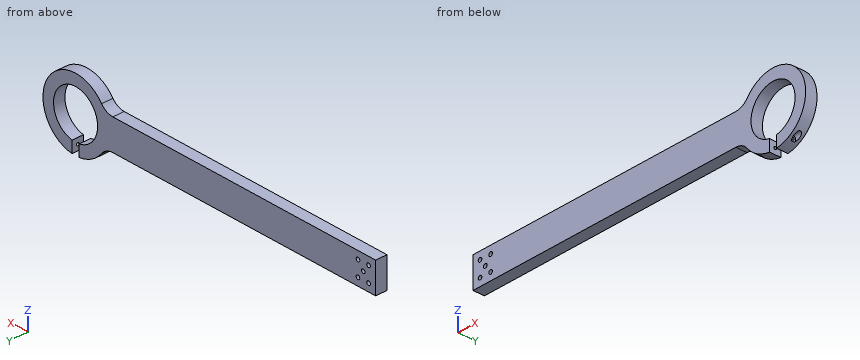
from build123d import *

# Parameters (mm, degrees)
BOSS_EXTRUDE1_DEPTH   = 4.7625
SKETCH8_W             = 1.1303
SKETCH8_H             = 266.825
F_4_40_TAPPED_HOLE2_D = 2.2606
FILLET2_R             = 12.7
CUT_EXTRUDE1_START    = -9.525
SKETCH11_R            = 2.413
CUT_EXTRUDE1_DEPTH    = 17.6497001
F_4_CLEARANCE_HOLE1_D = 3.2639


with BuildPart() as part:
    # Sketch2 → Boss-Extrude1 (new body, symmetric)
    with BuildSketch(Plane(origin=(0, 0, 0), x_dir=(1, 0, 0), z_dir=(0, 1, 0))):
        with BuildLine():
            Line((266.825, 19.568804386), (266.825, 29.177461594))
            ThreePointArc((266.825, 29.177461594), (253.046230135, 23.957766537), (243.54031576, 12.7))
            Line((243.54031576, 12.7), (0, 12.7))
            Line((0, 12.7), (0, -12.7))
            Line((0, -12.7), (243.54031576, -12.7))
            ThreePointArc((243.54031576, -12.7), (293.957766537, -16.953769865), (273.175, 29.177461594))
            Line((273.175, 29.177461594), (273.175, 19.568804386))
            ThreePointArc((273.175, 19.568804386), (270, -19.8247), (266.825, 19.568804386))
        make_face()
    extrude(amount=BOSS_EXTRUDE1_DEPTH, both=True)

    # Sketch8 → #4-40 Tapped Hole1 (revolve, cut)
    with BuildSketch(Plane(origin=(266.825, 0, -24.37313299), x_dir=(0, 0, -1), z_dir=(0, 1, 0))):
        with Locations((0.56515, 133.4125)):
            Rectangle(SKETCH8_W, SKETCH8_H)
    revolve(axis=Axis((273.175, 0, -24.37313299), (-1, 0, 0)), mode=Mode.SUBTRACT)

    # #4-40 Tapped Hole2 (through all)
    with Locations(Plane.ZY.offset(-273.175)):
        with Locations((-24.37313299, 0)):
            Hole(F_4_40_TAPPED_HOLE2_D / 2)

    # Fillet2
    fillet2_edges = [part.edges().sort_by_distance(p)[0] for p in [
        (243.54031576, 0, -12.7),
        (243.54031576, 0, 12.7),
    ]]
    fillet(fillet2_edges, radius=FILLET2_R)

    # Sketch11 → Cut-Extrude1 (cut, through all)
    with BuildSketch(Plane.ZY.offset(-273.175).offset(CUT_EXTRUDE1_START)):
        with Locations((-24.37313299, 0)):
            Circle(SKETCH11_R)
    extrude(amount=-CUT_EXTRUDE1_DEPTH, mode=Mode.SUBTRACT)

    # #4 Clearance Hole1 (through all)
    with Locations(Plane(origin=(0, -4.7625, 0), x_dir=(-1, 0, 0), z_dir=(0, -1, 0))):
        with Locations((-6.35, -6.35), (-15.875, 6.35), (-15.875, -6.35), (-11.1125, 0), (-6.35, 6.35)):
            Hole(F_4_CLEARANCE_HOLE1_D / 2)


solid = part.part
Source: CAD feature listing. Evaluate the final solid. Frame: model axes, mm. Coordinates: 2 decimals unless noted, no trailing zeros. Loops run counter-clockwise (first coordinate to the right, second up) from the corner with the lowest first, then second, coordinate; pieces in that order, holes last. Notation, with made-up numbers: (82.25, 51.25) - (128.25, 51.25) arc R26 ccw to (128.25, 75.25) - close; hole circle Ø2 at (32.25, 77). An arc over 180 degrees is marked (long way). One line per question, with ' | ' between items.
1) Section B-B, the plane x = 142. Return loops of the section in (y, z), then the cut area to 3 significant figures.
Report:
outline: (-4.76, -12.7) - (4.76, -12.7) - (4.76, 12.7) - (-4.76, 12.7) - close | area: 242 mm²
2) First-contact query: P1, Ø2, axis at y = 1, z = -23.5, coming from the +X side; P2, Ø3, axis at y = 0, z = -24.37, coming from the -X side; P3, Ø1, axis at y = -2, z = -7.5, coming from the +X side. Flat tips, straight axial feed; report the tip coordinate or a pass-through.
Report:
P1: stops at x = 282.7 | P2: stops at x = 251.61 | P3: stops at x = 298.5
3) Section A-A, the plane x = 270. Return loops of the section in (y, z).
Report:
outline: (-4.76, 19.82) - (4.76, 19.82) - (4.76, 29.35) - (-4.76, 29.35) - close
4) Line query: line 1 along Z through (x, y) = (6.35, -0.25); line 2 along X through (y, z) = (-2.25, -6.35); line 3 along Z through (x, y) = (13, -1.5). Output: solid intervals per line, ascending.
Report:
line 1: z = -12.7 to -7.98, -4.72 to 4.72, 7.98 to 12.7 | line 2: x = 0 to 4.72, 7.98 to 14.24, 17.51 to 251.22, 288.78 to 298.65 | line 3: z = -12.7 to 12.7
